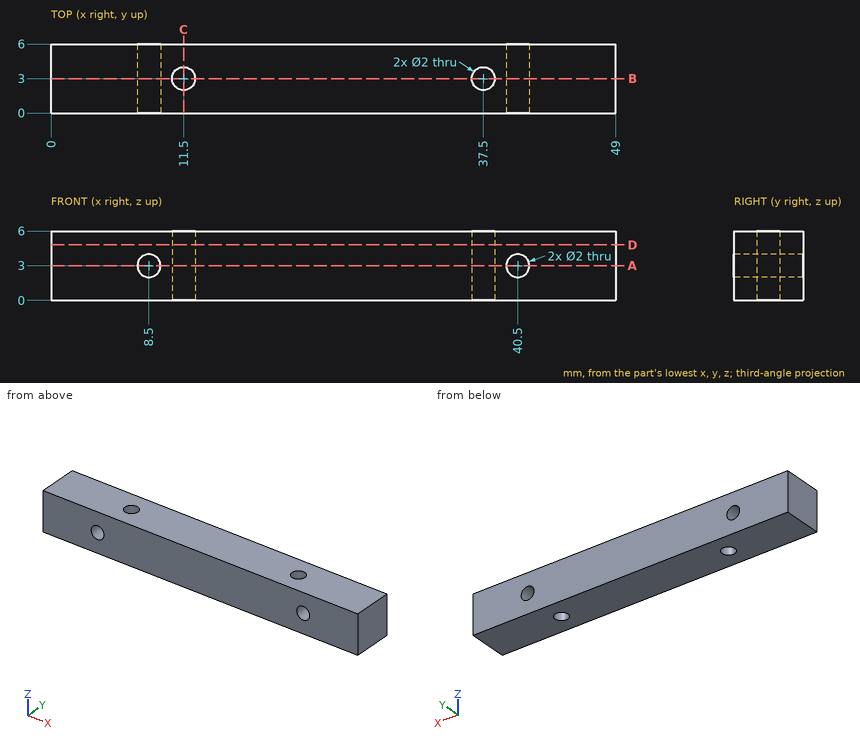
Geometry: see drawing. Coordinates: mm, zero at the bounding-box minimum. Give positions to 0.01 mm unless a question says otherwise; leave off trailing zeros. Write each loop counter-clockwise with the first axis right and the second up, starting at its lowest first coordinate (ties: lowest second). Pieces come first, ordered by that corner, then holes. Notation, with made-up numbers: M 66.5,-19.75 L 88.5,-19.75 A20 ccw 88.5,6.25 Z; hole C 23,36.5 d3. An arc over 180 degrees is marked long. Return JSON: item names as keys, results as strings. Group by question number.
1) Cut plane A-A, the plane z = 3. Output: boundary loops of the cut face in (x, y), then the cut area to 3 significant figures.
2) Cut plane B-B, the plane y = 3. Output: boundary loops of the cut face in (x, z).
3) Cut plane C-C, the plane x = 11.5. Output: boundary loops of the cut face in (y, z), then the cut area to 3 significant figures.
4) Ray query, L1, parallel to X at y = 4.1, z = 3; L2, parallel to Y at x = 37.5, z = 4.4; L3, parallel to X at y = 3, z = 3.45. Return the intervals inside material, ascending.
5) First-contact query: pin 1 Ø1.8 at (x, y) = (37.5, 3) entering from +Z. Flat tip, straight axial feed; report the tip coordinate or a pass-through.
6) Cut plane D-D, the plane z = 4.8. Output: boundary loops of the cut face in (x, y).
Data:
{
 "1": {"outline": "M 0,0 L 7.5,0 L 7.5,6 L 0,6 Z; M 9.5,0 L 39.5,0 L 39.5,6 L 9.5,6 Z; M 41.5,0 L 49,0 L 49,6 L 41.5,6 Z; hole C 11.5,3 d2; hole C 37.5,3 d2", "area": "264 mm²"},
 "2": {"outline": "M 0,0 L 10.5,0 L 10.5,6 L 0,6 Z; M 12.5,0 L 36.5,0 L 36.5,6 L 12.5,6 Z; M 38.5,0 L 49,0 L 49,6 L 38.5,6 Z; hole C 8.5,3 d2; hole C 40.5,3 d2"},
 "3": {"outline": "M 0,0 L 2,0 L 2,6 L 0,6 Z; M 4,0 L 6,0 L 6,6 L 4,6 Z", "area": "24.0 mm²"},
 "4": {"L1": "x = 0 to 7.5, 9.5 to 39.5, 41.5 to 49", "L2": "y = 0 to 2, 4 to 6", "L3": "x = 0 to 7.61, 9.39 to 10.5, 12.5 to 36.5, 38.5 to 39.61, 41.39 to 49"},
 "5": {"pin 1": "passes through"},
 "6": {"outline": "M 0,0 L 49,0 L 49,6 L 0,6 Z; hole C 11.5,3 d2; hole C 37.5,3 d2"}
}
